Autodesk Inventor part; units mm, degrees
ref_plane "YZ Plane" through (0, 0, 0) normal (1, 0, 0) x (0, 1, 0)
ref_plane "XZ Plane" through (0, 0, 0) normal (0, 1, 0) x (-1, 0, 0)
ref_plane "XY Plane" through (0, 0, 0) normal (0, 0, 1) x (1, 0, 0)
sketch "Sketch1" plane through (0, 0, 0) normal (0, 1, 0) x (-1, 0, 0)
  circle A0 centre (0, 0) radius 4.95
  dimension "d0" = 9.9
extrude "Extrusion1" add sketch "Sketch1" along normal blind 8
sketch "Sketch2" plane through (0, 8, 0) normal (0, 1, 0) x (1, 0, 0)
  circle A0 centre (0, 0) radius 2.4
  line L0 (-0.65, -3.9) -> (0.65, -3.9)
  line L1 (0.65, -3.9) -> (0.65, 3.9)
  line L2 (0.65, 3.9) -> (-0.65, 3.9)
  line L3 (-0.65, 3.9) -> (-0.65, -3.9)
  line L4 (-0.65, -3.9) -> (0.65, 3.9) construction
  line L5 (0.65, -3.9) -> (-0.65, 3.9) construction
  point P0 (-0.65, 2.3103)
  point P1 (-0.65, -2.3103)
  point P2 (0.65, -2.3103)
  point P3 (0.65, 2.3103)
  dimension "d3" = 4.8
  dimension "d4" = 1.3
  dimension "d5" = 7.8
extrude "Extrusion2" add sketch "Sketch2" along normal blind 24
sketch "Sketch3" plane through (0, 0, 0) normal (0, -1, 0) x (1, 0, 0)
  circle A0 centre (0, 0) radius 3
  dimension "d8" = 6
extrude "Extrusion3" add sketch "Sketch3" along normal blind 5
sketch "Sketch4" plane through (0, -5, 0) normal (0, -1, 0) x (1, 0, 0)
  arc A0 (-0.65, 2.3103) -> (-0.65, -2.3103) centre (0, 0) ccw
  circle A1 centre (0, 0) radius 1.75
  line L0 (1.3857, -0.85) -> (-1.5, -0.85)
  line L1 (1.3857, -0.85) -> (1.8275, -0.85)
  line L2 (-1.5, -0.85) -> (-1.5752, -0.85)
  point P0 (-0.5831, -1.65)
  point P1 (0.5831, -1.65)
  point P2 (1.5297, -0.85)
  point P3 (-1.5297, -0.85)
  dimension "d11" = 3.5
  dimension "d12" = 2.6
extrude "Extrusion6" cut sketch "Sketch4" against normal blind 10 contours A1 L1 L0 L2 picked at (-0.5593, -0.3047)
properties part number "spojkaMotoruSRotorem"
Geometry: final body of the model. Coordinates: model frame, mm. A direction names the side the tool comes from. Coordinates: 2 decimals unless noted, no trailing zeros. Order: outer loops, then holes, each group sorted by start corner. A loop starts at its lowest first (then second) coordinate and runs counter-clockwise, first axis right, second up. Notation, with made-up numbers: (18.25, 25) - (37.25, 25) arc R14 ccw to (37.25, 34) - close; hole circle Ø8 at (78, 61). An arc over 180 degrees is marked (long way). Return JSON: item names as keys, results as strings. Group by question number.
1. Cut plane B-B (x = 0). Output: boundary loops of the cut face in (y, z).
2. Pull-direction query (X, two-part tool) for faces 1 (the face through (0, 5, 0)), 2 (the face through (0, 32, 0)), 3 (the face through (0.65, 20, -3)); classes: pulls with the +X half, pulls with the -X half, needs draft (parallel to the pull), parting line crosses it, or undercut.
3. Material intervals for line 1 along Z through (x, y) = (0, -0.75); line 2 along Z through (x, y) = (0, 0.5); line 3 along X through (y, z) = (21, 0), sorted ascending. Write a range as [from, to].
4. Cut plane C-C (y = 17). Output: boundary loops of the cut face in (x, z).
5. Set-up query: faces 4 (the face through (-2.4, 19.8, 0)), 5 (the face through (-0.65, 20, 3)), 6 (the face through (0, 20, -3.9)), 7 (the face through (0, 20, 3.9)), 8 (the face through (-3, -2, 0)). Return all of +Z, -Z, +X, -X, +Y, -Y with unobstructed straight access to the full face (end or side cutting, diameter ignored); none if empty.
6. Cut plane A-A (z = 0). Output: boundary loops of the cut face in (x, y), plus the area to 3 significant figures.
7. Pin query (flat end, axial travel): pin 1 (4 mm diameter, centred on y = 24.5, z = 1.5, fed in from -X); pin 2 (1.5 mm diameter, centred on y = 25.5, z = 1.5, fed in from +X); pin 3 (0.8 mm diameter, centred on y = 25.5, z = 3.5, fed in from +X). Return the tip coordinate at first contact, or that it passes through.
8. Cut plane D-D (y = 3.5). Output: boundary loops of the cut face in (x, z).
Resolved:
{
 "1": {"outline": "(-5, -3) - (0, -3) - (0, -4.95) - (8, -4.95) - (8, -3.9) - (32, -3.9) - (32, 3.9) - (8, 3.9) - (8, 4.95) - (0, 4.95) - (0, 3) - (-5, 3) - (-5, 1.75) - (5, 1.75) - (5, -0.85) - (-5, -0.85) - close"},
 "2": {"face 1": "undercut", "face 2": "needs draft", "face 3": "pulls with the +X half"},
 "3": {"line 1": "z = [-3, -0.85], [1.75, 3]", "line 2": "z = [-4.95, -0.85], [1.75, 4.95]", "line 3": "x = [-2.4, 2.4]"},
 "4": {"outline": "(-0.65, -3.9) - (0.65, -3.9) - (0.65, -2.31) arc R2.4 ccw to (0.65, 2.31) - (0.65, 3.9) - (-0.65, 3.9) - (-0.65, 2.31) arc R2.4 ccw to (-0.65, -2.31) - close"},
 "5": {"face 4": "-X, +Y", "face 5": "+Z, -X, +Y", "face 6": "-Z, +X, -X, +Y", "face 7": "+Z, +X, -X, +Y", "face 8": "-Y"},
 "6": {"outline": "(-4.95, 0) - (-3, 0) - (-3, -5) - (-1.75, -5) - (-1.75, 5) - (1.75, 5) - (1.75, -5) - (3, -5) - (3, 0) - (4.95, 0) - (4.95, 8) - (2.4, 8) - (2.4, 32) - (-2.4, 32) - (-2.4, 8) - (-4.95, 8) - close", "area": "189 mm²"},
 "7": {"pin 1": "stops at x = -2.4", "pin 2": "stops at x = 2.28", "pin 3": "stops at x = 0.65"},
 "8": {"outline": "circle Ø9.9 at (0, 0); hole (-1.53, -0.85) - (1.53, -0.85) arc R1.75 ccw (long way) to start"}
}
